Model file for the job. Use its own axes, mm. Give positions to 0.01 mm unless a question says otherwise; leave off trailing zeros. Order: outer loops, then holes, each group sorted by start corner. A loop starts at its lowest first (then second) coordinate and runs counter-clockwise, first axis right, second up. Notation, with made-up numbers: (-34.5, 0.5) - (24.5, 0.5) arc R14 cw to (24.5, 18.5) - close; hole circle Ø5 at (-15, 84). An arc over 180 degrees is marked (long way). Use CSV: the item, a comma, the result in double quotes. Start each with the question number.
(1) Band-saw the part on A-A, the plane x = 0. Give the cut face in (y, z).
(2) Band-saw the part on C-C, the plane z = 38. Give the cut face in (x, y).
(3) Probe L1, parallel to X at y = 0, z = -4; L2, parallel to Z at x = -3.75, y = 2.5; L3, parallel to X at y = -1.5, z = 21.5. List the from-to ranges inside material, lowest first.
(4) Drop flat-ended pins along their axis: pin 1 Ø1.5 at (y, z) = (-3.5, 1.5) entering from -X; pin 2 Ø2 at (y, z) = (-3.5, -43) entering from +X; pin 3 Ø4.5 at (x, y) = (0, 0) entering from +Z. Give the stop position or say it passes through.
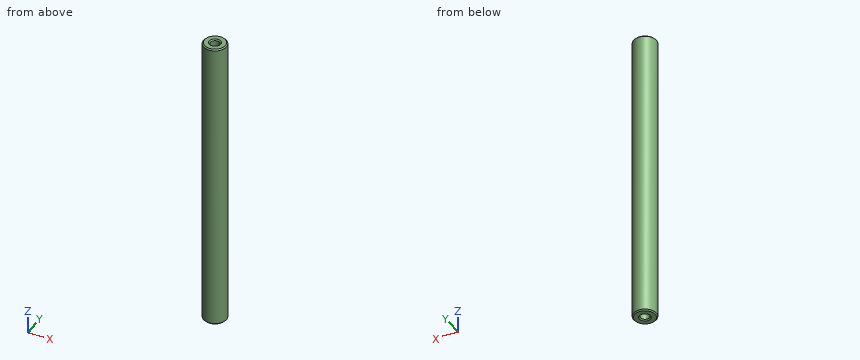
Autodesk Inventor part; units mm, degrees
ref_plane "YZ Plane" through (0, 0, 0) normal (1, 0, 0) x (0, 1, 0)
ref_plane "XZ Plane" through (0, 0, 0) normal (0, 1, 0) x (-1, 0, 0)
ref_plane "XY Plane" through (0, 0, 0) normal (0, 0, 1) x (1, 0, 0)
sketch "Boceto1" plane through (0, 0, 0) normal (1, 0, 0) x (0, 1, 0)
  line L0 (0, 65) -> (0, -65) construction
  line L1 (2, 65) -> (5, 65)
  line L2 (5, 65) -> (5, -65)
  line L3 (5, -65) -> (2, -65)
  line L4 (2, -65) -> (2, 65)
  point P0 (0, 0)
  point P1 (0, 0)
  dimension "d0" = 130
  dimension "d1" = 10
  dimension "d2" = 3
revolve "Revolución1" add sketch "Boceto1" angle 360 about axis through (0, 0, 65) along (0, 0, -1)
thread "Rosca1"
chamfer "Chaflán1" distance 0.5 angle 45 4 edges at (0, -2, 65) (0, -5, 65) (0, -2, -65) (0, -5, -65)
properties part number "eje_manzana_delantera"
Answer block:
1,outline,"(-5, -64.5) - (-4.5, -65) - (-2.5, -65) - (-2, -64.5) - (-2, 64.5) - (-2.5, 65) - (-4.5, 65) - (-5, 64.5) - close; (2, -64.5) - (2.5, -65) - (4.5, -65) - (5, -64.5) - (5, 64.5) - (4.5, 65) - (2.5, 65) - (2, 64.5) - close"
2,outline,"circle Ø10 at (0, 0); hole circle Ø4 at (0, 0)"
3,L1,"x = -5 to -2, 2 to 5"
3,L2,"z = -64.99 to 64.99"
3,L3,"x = -4.77 to -1.32, 1.32 to 4.77"
4,pin 1,"stops at x = -4.18"
4,pin 2,"stops at x = 4.33"
4,pin 3,"stops at z = 64.75"
